Autodesk Inventor part; units mm, degrees
ref_plane "YZ Plane" through (0, 0, 0) normal (1, 0, 0) x (0, 1, 0)
ref_plane "XZ Plane" through (0, 0, 0) normal (0, 1, 0) x (-1, 0, 0)
ref_plane "XY Plane" through (0, 0, 0) normal (0, 0, 1) x (1, 0, 0)
sketch "Sketch1" plane through (0, 0, 0) normal (0, 0, 1) x (1, 0, 0)
  line L0 (0, 0) -> (25.4, 0)
  line L1 (25.4, 0) -> (25.4, 76.2)
  line L2 (25.4, 76.2) -> (0, 76.2)
  line L3 (0, 76.2) -> (0, 0)
  line L4 (0, 76.2) -> (76.2, 76.2)
  line L5 (76.2, 76.2) -> (76.2, 50.8)
  line L6 (76.2, 50.8) -> (0, 50.8)
  line L7 (0, 50.8) -> (0, 76.2)
  dimension "d0" = 25.4
  dimension "d1" = 76.2
  dimension "d2" = 76.2
  dimension "d3" = 25.4
extrude "Extrusion1" add sketch "Sketch1" along normal blind 3.175
sketch "Sketch2" plane through (0, 0, 3.175) normal (0, 0, 1) x (1, 0, 0)
  line L0 (0, 0) -> (25.4, 0) construction
  line L1 (12.7, 0) -> (12.7, 12.7) construction
  line L2 (12.7, 12.7) -> (12.7, 38.1) construction
  line L3 (12.7, 38.1) -> (12.7, 63.5) construction
  line L4 (12.7, 63.5) -> (38.1, 63.5) construction
  line L5 (38.1, 63.5) -> (63.5, 63.5) construction
  circle A0 centre (63.5, 63.5) radius 2.5797
  circle A1 centre (38.1, 63.5) radius 2.5797
  circle A2 centre (12.7, 63.5) radius 2.5797
  circle A3 centre (12.7, 38.1) radius 2.5797
  circle A4 centre (12.7, 12.7) radius 2.5797
  dimension "d6" = 12.7
  dimension "d7" = 25.4
  dimension "d8" = 25.4
  dimension "d11" = 25.4
  dimension "d12" = 25.4
  dimension "d13" = 5.1594
extrude "Extrusion2" cut sketch "Sketch2" against normal blind 3.175
fillet "Fillet1" radius 3.175 6 edges at (76.2, 76.2, 1.5875) (0, 76.2, 1.5875) (76.2, 50.8, 1.5875) (25.4, 50.8, 1.5875) (25.4, 0, 1.5875) (0, 0, 1.5875)
properties part number "0.125 L-Gusset"
For this review, take the finished solid that the model builds, in its own axes (mm). A direction names the side the tool comes from. Round coordinates to 2 decimals unless told otherwise and drop trailing zeros. Loops run counter-clockwise (first coordinate to the right, second up) from the corner with the lowest first, then second, coordinate; pieces in that order, holes last. Notation, with made-up numbers: (-39.5, -21.5) - (14.5, -21.5) arc R19 cw to (14.5, -1.5) - close; hole circle Ø3 at (-5, 42.5). An arc over 180 degrees is marked (long way). Answer as CSV lines item,"result".
(1) Wall thickness on line 1 (Y direction, x = 12.7, z = 0.7); line 2 (X direction, y = 61.5, z = 1.75); line 3 (Y direction, x = 63.5, z = 2.1): over which ranges is each line inside the solid? List them lowest first.
Checked values:
line 1,"y = 0 to 10.12, 15.28 to 35.52, 40.68 to 60.92, 66.08 to 76.2"
line 2,"x = 0 to 11.07, 14.33 to 36.47, 39.73 to 61.87, 65.13 to 76.2"
line 3,"y = 50.8 to 60.92, 66.08 to 76.2"
(2) Consider section D-D on y = 24.5. Give the boundary of the cut face in (x, z) (3 decimals), then the cut area to 3 significant figures.
Checked values:
outline,"(0, 0) - (25.4, 0) - (25.4, 3.175) - (0, 3.175) - close"
area,"80.6 mm2"
(3) Mouldability with a two-part tool opening along Y and no side actions: class faces 3 (the face through (51, 50.8, 2)), 4 (the face through (75.29, 75.25, 1.61)), 5 (the face through (12.364, 66.058, 1.61)) as +Y half, -Y half, draft (parallel to the pull), parting line (faces both ways), or undercut.
Checked values:
face 3,"-Y half"
face 4,"+Y half"
face 5,"undercut"
(4) Tool access review of faces 1 (the face through (0.91, 0.95, 1.61)), 2 (the face through (25.4, 25, 2)): name each direction out of +Z, -Z, +X, -X, +Y, -Y from which nothing blocks a thin tool from reaching the whole face with its end or side.
Checked values:
face 1,"+Z, -Z, -X, -Y"
face 2,"+Z, -Z, +X, -Y"
(5) Consider section B-B on y = 12.7. Give the boundary of the cut face in (x, z) (3 decimals), then the cut area to 3 significant figures.
Checked values:
outline,"(0, 0) - (10.12, 0) - (10.12, 3.175) - (0, 3.175) - close; (15.28, 0) - (25.4, 0) - (25.4, 3.175) - (15.28, 3.175) - close"
area,"64.3 mm2"
(6) Insertion check: P1, Ø1, axis at y = 31, z = 2.5, coming from the +X side; P2, Ø8.5, axis at x = 63.5, y = 63.5, coming from the -Z side; P3, Ø1.6, axis at x = 54, z = 2.5, coming from the -Y side. Each pin has a flat end and moves straight along its axis. Give the tip position at first contact, or say it passes through.
Checked values:
P1,"stops at x = 25.4"
P2,"stops at z = 0"
P3,"stops at y = 50.8"
(7) Consider section A-A on x = 38.1. Give the boundary of the cut face in (y, z) (3 decimals).
Checked values:
outline,"(50.8, 0) - (60.92, 0) - (60.92, 3.175) - (50.8, 3.175) - close; (66.08, 0) - (76.2, 0) - (76.2, 3.175) - (66.08, 3.175) - close"
(8) Consider section C-C on z = 1.05. Give the boundary of the cut face in (x, y) (3 decimals), then the cut area to 3 significant figures.
Checked values:
outline,"(0, 3.175) arc R3.175 ccw to (3.175, 0) - (22.225, 0) arc R3.175 ccw to (25.4, 3.175) - (25.4, 47.625) arc R3.175 cw to (28.575, 50.8) - (73.025, 50.8) arc R3.175 ccw to (76.2, 53.975) - (76.2, 73.025) arc R3.175 ccw to (73.025, 76.2) - (3.175, 76.2) arc R3.175 ccw to (0, 73.025) - close; hole circle Ø5.159 at (12.7, 12.7); hole circle Ø5.159 at (12.7, 38.1); hole circle Ø5.159 at (12.7, 63.5); hole circle Ø5.159 at (38.1, 63.5); hole circle Ø5.159 at (63.5, 63.5)"
area,"3,110 mm2"
